Autodesk Inventor part; units mm, degrees
ref_plane "YZ Plane" through (0, 0, 0) normal (1, 0, 0) x (0, 1, 0)
ref_plane "XZ Plane" through (0, 0, 0) normal (0, 1, 0) x (-1, 0, 0)
ref_plane "XY Plane" through (0, 0, 0) normal (0, 0, 1) x (1, 0, 0)
sketch "Sketch1" plane through (0, 0, 0) normal (0, 1, 0) x (-1, 0, 0)
  circle A0 centre (0, 0) radius 2.5
  dimension "d0" = 5
extrude "Extrusion1" add sketch "Sketch1" along normal blind 20
sketch "Sketch2" plane through (0, 20, 0) normal (0, 1, 0) x (1, 0, 0)
  circle A0 centre (0, 0) radius 1.25
  dimension "d3" = 2.5
extrude "Extrusion2" add sketch "Sketch2" along normal blind 6
sketch "Sketch3" plane through (0, 0, 0) normal (0, -1, 0) x (1, 0, 0)
  circle A0 centre (0, 0) radius 1.25
  dimension "d6" = 2.5
extrude "Extrusion3" cut sketch "Sketch3" against normal blind 6
thread "Thread1"
thread "Thread2"
properties part number "Mock Spacer"
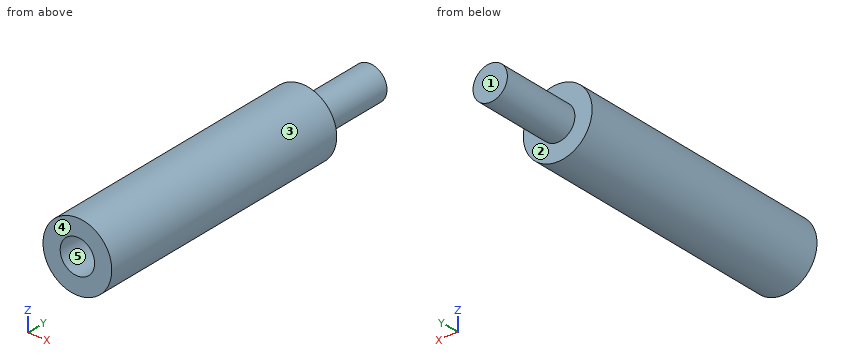
Part model, mm, in its own coordinate system. Face numbers are marked on the shaded views. A direction names the side the tool comes from. Coordinates: 2 decimals unless noted, no trailing zeros. Loops run counter-clockwise (first coordinate to the right, second up) from the corner with the lowest first, then second, coordinate; pieces in that order, holes last. Notation, with made-up numbers: (35.25, 48) - (40.25, 48) arc R21 ccw to (40.25, 58) - close; hole circle Ø11 at (18.25, 60.5). An arc over 180 degrees is marked (long way). Write each question's results on one line, items separated by ' | '. Start each with the question number.
Q1. Slice it at D-D on y = 24.5. Give the cut face in (x, z), and give its area (3 significant figures).
Q2. Two-plate mould, pull along X, no slides. Class the marked faces 3, 4 and 5: +X half, -X half, draft (parallel to the pull), parting line (faces both ways), or undercut.
Q3. Slice it at A-A on z = 0. Give the cut face in (x, y).
Q4. Slice it at B-B on x = 0. Give the cut face in (y, z).
Q5. Drop flat-ended pins along their axis: pin 1 Ø1.5 at (x, z) = (1.5, -1) entering from +Y; pin 2 Ø0.8 at (x, z) = (0, -0.5) entering from -Y; pin 3 Ø1 at (y, z) = (10, -2) entering from +X. Give the stop position or say it passes through.
Q6. Probe line 1 along Z through (x, y) = (0, 2.6); line 2 along Y through (x, z) = (0.95, -0.25); line 3 along Y through (x, z) = (-2, -0.1). List the from-to ranges inside material, lowest first.
Q7. Slice it at C-C on y = 5.25. Give the cut face in (x, z), and give its area (3 significant figures).
Q8. Which spindle directions (+Z, -Z, +X, -X, +Y, -Y) get a long thin tool onto all of the face, cutting with end or side? Do the marked faces 1 and 2. Say none if no direction does.
Answer:
1) outline: circle Ø2.5 at (0, 0) | area: 4.91 mm2
2) face 3: parting line | face 4: draft | face 5: undercut
3) outline: (-2.5, 0) - (-1.25, 0) - (-1.25, 6) - (1.25, 6) - (1.25, 0) - (2.5, 0) - (2.5, 20) - (1.25, 20) - (1.25, 26) - (-1.25, 26) - (-1.25, 20) - (-2.5, 20) - close
4) outline: (0, -2.5) - (20, -2.5) - (20, -1.25) - (26, -1.25) - (26, 1.25) - (20, 1.25) - (20, 2.5) - (0, 2.5) - (0, 1.25) - (6, 1.25) - (6, -1.25) - (0, -1.25) - close
5) pin 1: stops at y = 26 | pin 2: stops at y = 6 | pin 3: stops at x = 2
6) line 1: z = -2.5 to -1.25, 1.25 to 2.5 | line 2: y = 6 to 26 | line 3: y = 0 to 20
7) outline: circle Ø5 at (0, 0); hole circle Ø2.5 at (0, 0) | area: 14.7 mm2
8) face 1: +Z, -Z, +X, -X, +Y | face 2: +Y
